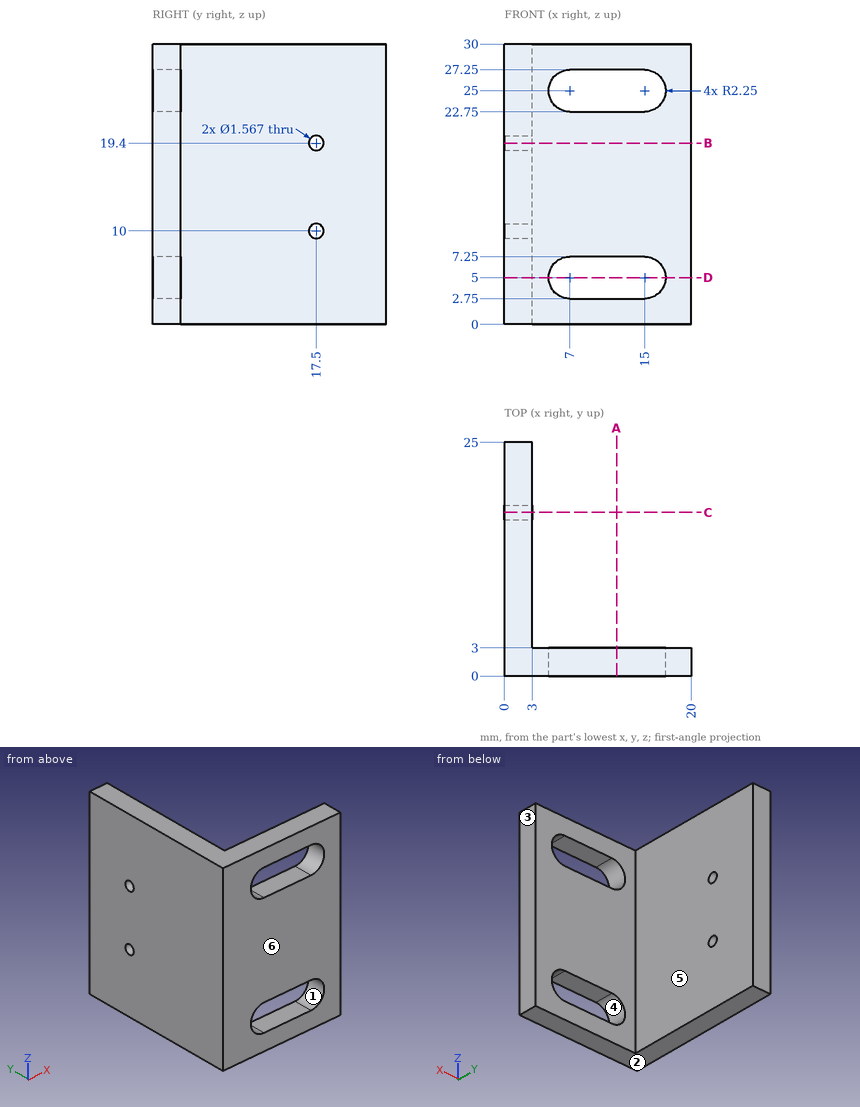
Study the drawing (mm; zero at the part's minimum x, y, z) and answer. A direction names the side the tool comes from. Round coordinates to 2 decimals unless told otherwise and drop trailing zeros. Loops run counter-clockwise (first coordinate to the right, second up) from the corner with the lowest first, then second, coordinate; pieces in that order, holes last. Notation, with made-up numbers: (-11.5, 89.5) -> (16.5, 89.5) arc R10 ccw to (16.5, 99.5) -> close; hole circle Ø3 at (-37, -17). An arc over 180 degrees is marked (long way). One line per item, written item: value.
1) A cutting plane is placed at D-D (z = 5). Determine the outline of the cut face in (x, y), and give its area (3 significant figures).
Answer list:
outline: (0, 0) -> (4.75, 0) -> (4.75, 3) -> (3, 3) -> (3, 25) -> (0, 25) -> close; (17.25, 0) -> (20, 0) -> (20, 3) -> (17.25, 3) -> close
area: 88.5 mm²
2) Flat-ended cylindrical pins translate along their axes: P1, Ø3, axis at x = 16.5, z = 24, coming from the +Y side; P2, Ø2, axis at y = 17.5, z = 19.4, coming from the +X side. Find the tip coordinate at first contact, or state that the pin passes through.
Answer list:
P1: stops at y = 3
P2: stops at x = 3
3) A cutting plane is placed at C-C (y = 17.5). Determine the outline of the cut face in (x, z), and give its area (3 significant figures).
Answer list:
outline: (0, 0) -> (3, 0) -> (3, 9.22) -> (0, 9.22) -> close; (0, 10.78) -> (3, 10.78) -> (3, 18.62) -> (0, 18.62) -> close; (0, 20.18) -> (3, 20.18) -> (3, 30) -> (0, 30) -> close
area: 80.6 mm²
4) A cutting plane is placed at B-B (z = 19.4). Determine the outline of the cut face in (x, y).
Answer list:
outline: (0, 0) -> (20, 0) -> (20, 3) -> (3, 3) -> (3, 16.72) -> (0, 16.72) -> close; (0, 18.28) -> (3, 18.28) -> (3, 25) -> (0, 25) -> close
5) The mould has two halves that part along Z. Classify the marked faces 1, 2 and 3: pulls with the +Z half, pulls with the -Z half, needs draft (parallel to the pull), parting line crosses it, or undercut.
Answer list:
face 1: undercut
face 2: pulls with the -Z half
face 3: needs draft
6) A cutting plane is placed at A-A (x = 12). Determine the outline of the cut face in (y, z), and give its area (3 significant figures).
Answer list:
outline: (0, 0) -> (3, 0) -> (3, 2.75) -> (0, 2.75) -> close; (0, 7.25) -> (3, 7.25) -> (3, 22.75) -> (0, 22.75) -> close; (0, 27.25) -> (3, 27.25) -> (3, 30) -> (0, 30) -> close
area: 63.0 mm²
7) Consider L1, parallel to Z at x = 1, y = 17.5; L2, parallel to Y at x = 2, z = 10; L3, parallel to Z at x = 8.5, y = 2.5. Determine where each line is inside the solid, lowest interval first. Write a range as [from, to].
Answer list:
L1: z = [0, 9.22], [10.78, 18.62], [20.18, 30]
L2: y = [0, 16.72], [18.28, 25]
L3: z = [0, 2.75], [7.25, 22.75], [27.25, 30]
8) For the marked faces 4, 5 and 6, determine the directions among +Z, -Z, +X, -X, +Y, -Y from which every point of the face is accessible in a straight line to the end or side of a thin tool.
Answer list:
face 4: +Y, -Y
face 5: +Z, -Z, +X, +Y
face 6: +Z, -Z, +X, -X, -Y
